Design review of the part built by this model. Coordinates are the model's own, in mm. Face numbers are marked on the shaded views. Coordinates: 2 decimals unless noted, no trailing zeros. Loops run counter-clockwise (first coordinate to the right, second up) from the corner with the lowest first, then second, coordinate; pieces in that order, holes last. Notation, with made-up numbers: M 82,-20.5 L 111,-20.5 A16 ccw 111,-5.5 Z; hole C 15.25,5.25 d9. An arc over 180 degrees is marked long. Answer as a JSON object with one key per item and string values. Group by question number.
1. Insertion check: pin 1 (0.9 mm diameter, centred on x = -16, z = 22, fed in from +Y); pin 2 (2.5 mm diameter, centred on x = 17, z = 22.5, fed in from +Y). Each pin has a flat end and moves straight along its axis. Give the tip position at first contact, or say it passes through.
2. Draft analysis for pull direction X (two halves, no side actions). For the marked faces 1, 2 and 3, state which applies: +X half, -X half, draft (parallel to the pull), parting line (faces both ways), or undercut.
3. Consider section A-A (x = -16.75). State the section outline as (y, z) points.
4. Consider section C-C (z = 4). State the section outline as (x, y) points, then the cut area to 3 significant figures.
5. To check wall thickness, follow probe 1 along X at (y, z) = (3, 22.25); probe 2 along Z at (x, y) = (-16.75, 8.25); probe 3 along Y at (x, z) = (16.5, 20.5). State the ranges of each line that lie inside material, in increasing order.
6. Consider section B-B (y = 12.75). State the section outline as (x, z) points.
7. Consider section D-D (x = 2). State the section outline as (y, z) points, then the cut area to 3 significant figures.
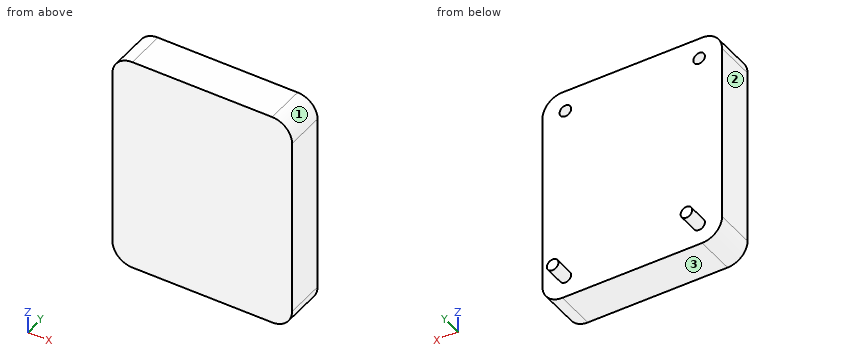
Autodesk Inventor part; units mm, degrees
ref_plane "YZ Plane" through (0, 0, 0) normal (1, 0, 0) x (0, 1, 0)
ref_plane "XZ Plane" through (0, 0, 0) normal (0, 1, 0) x (-1, 0, 0)
ref_plane "XY Plane" through (0, 0, 0) normal (0, 0, 1) x (1, 0, 0)
sketch "Esboço1" plane through (0, 0, 0) normal (0, 1, 0) x (-1, 0, 0)
  line L0 (-22.5, 27.5) -> (22.5, 27.5)
  line L1 (22.5, 27.5) -> (22.5, -27.5)
  line L2 (22.5, -27.5) -> (-22.5, -27.5)
  line L3 (-22.5, -27.5) -> (-22.5, 27.5)
  line L4 (-22.5, 27.5) -> (22.5, -27.5) construction
  line L5 (22.5, 27.5) -> (-22.5, -27.5) construction
  circle A0 centre (16.75, -22.25) radius 1.45
  circle A1 centre (16.75, 22.25) radius 1.45
  circle A2 centre (-16.75, 22.25) radius 1.45
  circle A3 centre (-16.75, -22.25) radius 1.45
  line L6 (-16.75, 22.25) -> (-16.75, -22.25) construction
  line L7 (-16.75, -22.25) -> (16.75, -22.25) construction
  line L8 (16.75, -22.25) -> (16.75, 22.25) construction
  line L9 (16.75, 22.25) -> (-16.75, 22.25) construction
  line L10 (0, 0) -> (9.1939, 0)
  line L11 (0, 0) -> (0, -6.5379)
  line L12 (16.75, 0) -> (30.08, 0) construction
  line L13 (0, 22.25) -> (0, 28.3312) construction
  dimension "d0" = 2.9
  dimension "d1" = 2.9
  dimension "d2" = 2.9
  dimension "d3" = 2.9
  dimension "d4" = 33.5
  dimension "d5" = 44.5
  dimension "d6" = 55
  dimension "d7" = 45
extrude "Extrusão1" add sketch "Esboço1" along normal blind 10 contours L0 L1 L2 L3 | A0 | A1 | A2 | A3
sketch "Esboço2" plane through (0, 10, 0) normal (0, 1, 0) x (1, 0, 0)
  circle A0 centre (16.75, -22.25) radius 1.45
  circle A1 centre (-16.75, -22.25) radius 1.45
  circle A2 centre (16.75, 22.25) radius 1.45
  circle A3 centre (-16.75, 22.25) radius 1.45
  point P0 (0, 0)
extrude "Extrusão2" cut sketch "Esboço2" against normal blind 8.5 contours A0 | A1
extrude "Extrusão3" add sketch "Esboço2" along normal blind 5 contours A2 | A3
fillet "Arredondamento1" radius 5 4 edges at (22.5, 5, 27.5) (22.5, 5, -27.5) (-22.5, 5, -27.5) (-22.5, 5, 27.5)
properties part number "BASE RELE"
Findings below:
{
 "1": {"pin 1": "stops at y = 1.5", "pin 2": "stops at y = 10"},
 "2": {"face 1": "+X half", "face 2": "-X half", "face 3": "draft"},
 "3": {"outline": "M 0,-27.5 L 10,-27.5 L 10,-23.7 L 15,-23.7 L 15,-20.8 L 10,-20.8 L 10,20.8 L 1.5,20.8 L 1.5,23.7 L 10,23.7 L 10,27.5 L 0,27.5 Z"},
 "4": {"outline": "M -22.5,0 L 22.5,0 L 22.5,10 L -22.5,10 Z", "area": "450 mm^2"},
 "5": {"probe 1": "x = -22.5 to -18.2, -15.3 to 15.3, 18.2 to 22.5", "probe 2": "z = -27.5 to 20.8, 23.7 to 27.5", "probe 3": "y = 0 to 10"},
 "6": {"outline": "C -16.75,-22.25 d2.9; C 16.75,-22.25 d2.9"},
 "7": {"outline": "M 0,-27.5 L 10,-27.5 L 10,27.5 L 0,27.5 Z", "area": "550 mm^2"}
}
